Autodesk Inventor part; units mm, degrees
ref_plane "YZ Plane" through (0, 0, 0) normal (1, 0, 0) x (0, 1, 0)
ref_plane "XZ Plane" through (0, 0, 0) normal (0, 1, 0) x (-1, 0, 0)
ref_plane "XY Plane" through (0, 0, 0) normal (0, 0, 1) x (1, 0, 0)
sketch "Skizze1" plane through (0, 0, 0) normal (1, 0, 0) x (0, 1, 0)
  line L0 (-10, -10) -> (-10, -5)
  line L1 (-10, -5) -> (-15, -5)
  line L2 (-15, -5) -> (-15, 0)
  line L3 (-15, 0) -> (15, 0)
  line L4 (15, 0) -> (15, -5)
  line L5 (15, -5) -> (10, -5)
  line L6 (10, -5) -> (10, -10)
  line L7 (10, -10) -> (20, -10)
  line L8 (20, -10) -> (20, -30)
  line L9 (20, -30) -> (-20, -30)
  line L10 (-20, -30) -> (-20, -10)
  line L11 (-20, -10) -> (-10, -10)
  line L12 (0, -36) -> (0, 6)
  point P0 (0, 0)
  dimension "d0" = 30
  dimension "d1" = 20
  dimension "d2" = 5
  dimension "d3" = 5
  dimension "d4" = 20
  dimension "d5" = 90
  dimension "d6" = 40
extrude "Extrusion1" add sketch "Skizze1" along normal blind 10
sketch "Skizze3" plane through (0, 20, -10) normal (0, 1, 0) x (1, 0, 0)
  line L0 (0, 0) -> (0, 20)
  line L1 (0, 20) -> (40, 20)
  line L2 (40, 20) -> (40, 80)
  line L3 (40, 80) -> (-10, 80)
  line L4 (-10, 80) -> (-10, 90)
  line L5 (-10, 90) -> (50, 90)
  line L6 (50, 90) -> (50, 10)
  line L7 (50, 10) -> (0, 10)
  point P0 (0, -10)
  dimension "d12" = 10
  dimension "d13" = 10
  dimension "d14" = 10
  dimension "d15" = 60
  dimension "d16" = 50
  dimension "d17" = 60
extrude "Extrusion3" add sketch "Skizze3" against normal up to surface (40 mm away)
sketch "Skizze4" plane through (50, 20, -100) normal (0, 0, -1) x (-1, 0, 0)
  arc A0 (53.3975, 30) -> (53.3975, -70) centre (140, -20) ccw
  arc A1 (62.0577, 25) -> (62.0577, -65) centre (140, -20) ccw
  line L0 (140, -20) -> (53.3975, -70)
  line L1 (140, -20) -> (53.3975, 30)
  line L2 (0, -40) -> (60, -40)
  line L3 (0, 0) -> (60, 0)
  line L4 (0, 0) -> (0, -40)
  point P0 (40, -20)
  point P1 (42.0204, 0)
  point P2 (52.2504, 0)
  point P3 (52.2504, -40)
  point P4 (42.0204, -40)
  dimension "d20" = 200
  dimension "d21" = 180
  dimension "d22" = 30
  dimension "d23" = 30
  dimension "d24" = 40
  dimension "d25" = 20
  dimension "d30" = 140
extrude "Extrusion4" add sketch "Skizze4" against normal up to surface (10 mm away) contours L1 A1 L3 A0 | L2 A1 L0 A0
sketch "Skizze5" plane through (40, -20, -90) normal (0, 0, 1) x (1, 0, 0)
  arc A0 (-42.2504, 40) -> (-52.0577, 65) centre (-130, 20) ccw
  circle A1 centre (-130, 20) radius 90
  point P0 (-40, 20)
  point P1 (-52.0577, 65)
  point P2 (-42.2504, 40)
extrude "Extrusion5" cut sketch "Skizze5" against normal up to surface (10 mm away)
sketch "Skizze6" plane through (40, -20, -90) normal (0, 0, 1) x (1, 0, 0)
  arc A0 (-52.0577, -25) -> (-52.0577, 65) centre (-130, 20) ccw
  line L0 (-43.3975, -30) -> (-52.0577, -25)
  arc A1 (-43.3975, -30) -> (-32.0204, 0) centre (-130, 20) ccw
  line L1 (-32.0204, 0) -> (0, 0)
  line L2 (0, 40) -> (0, 0)
  line L3 (-32.0204, 40) -> (0, 40)
  arc A2 (-32.0204, 40) -> (-43.3975, 70) centre (-130, 20) ccw
  line L4 (-52.0577, 65) -> (-43.3975, 70)
  line L5 (-30, 0) -> (-30, 40)
  line L6 (-30, 0) -> (10, 0)
  line L7 (10, 40) -> (10, 0)
  line L8 (-30, 40) -> (10, 40)
  point P0 (-40, 20)
extrude "Extrusion6" cut sketch "Skizze6" along normal through all
equation "\"d13\" = d12"
equation "\"d23\" = d22"
equation "\"d25\" = 0.5 * d24"
properties part number "Finger"
Could you check a few things on this model? Use its own coordinates, in mm. A direction names the side the tool comes from. Round coordinates to 2 decimals unless told otherwise and drop trailing zeros. Loops run counter-clockwise (first coordinate to the right, second up) from the corner with the lowest first, then second, coordinate; pieces in that order, holes last. Notation, with made-up numbers: M -6.75,48.5 L 42.25,48.5 A16 ccw 42.25,63.5 Z; hole C -34,21.5 d5. An arc over 180 degrees is marked long. Put each result on its own line as item: value.
Q1. I need wall thicknesses on probe 1 along Y at (x, z) = (31.5, -93); probe 2 along Y at (x, z) = (-7, -98.5); probe 3 along X at (y, z) = (-1, -93.75). Which ranges of each line are inside material? Lowest first, please.
Check result:
probe 1: -20 to 20
probe 2: -47.92 to -34.8, 34.8 to 47.92
probe 3: -0.01 to 50
Q2. Imagine slicing it at D-D (y = -3). Write out the boundary of the cut face in (x, z), then the cut area to 4 significant figures.
Check result:
outline: M -0.05,-100 L 50,-100 L 50,-90 L -0.05,-90 Z
area: 500.5 mm2
Q3. Imagine slicing it at C-C (x = 32.5). Write out the boundary of the cut face in (y, z).
Check result:
outline: M -20,-100 L 20,-100 L 20,-90 L -20,-90 Z
Q4. For pin 1 (4 mm diameter, centred on x = 32.5, z = -91.5, fed in from -Y); pin 2 (2 mm diameter, centred on y = 22.5, z = -94, fed in from -X), each with a flat end and sliding along its axis, tell me the tip position at first contact or that it passes through.
Check result:
pin 1: y = -20
pin 2: x = -3.12
Q5. Imagine slicing it at A-A (x = -6). Write out the boundary of the cut face in (y, z), then the cut area to 3 significant figures.
Check result:
outline: M -48.5,-100 L -32.31,-100 L -32.31,-90 L -48.5,-90 Z; M 32.31,-100 L 48.5,-100 L 48.5,-90 L 32.31,-90 Z
area: 324 mm2
Q6. Thinking about a two-plate mould opening in Y: for faces 4 (the face through (0, 0, -95)), 5 (the face through (29, 20, -95)), 6 (the face through (-7.788, -47.465, -95.07)), which applies, released by +Y, released by -Y, zero draft, split by the parting line, or undercut?
Check result:
face 4: undercut
face 5: released by +Y
face 6: released by -Y
Q7. Imagine slicing it at B-B (z = -94.5). Write out the boundary of the cut face in (x, y), then the cut area to 3 significant figures.
Check result:
outline: M -12.06,-45 L -3.4,-50 A100 ccw 7.98,-20 L 50,-20 L 50,20 L 7.98,20 A100 ccw -3.4,50 L -12.06,45 A90 cw Z
area: 2,620 mm2
Q8. On a 3-axis mill with a long thin cutter (end or side, diameter ignored), from which of +Z, -Z, +X, -X, +Y, -Y can I reach the whole of each face in a straight line? I mean faces 1 (the face through (-6.148, -32.692, -95.07)), 2 (the face through (29, -20, -95)), 3 (the face through (-7.788, 47.465, -95.07)). Say none if no direction works.
Check result:
face 1: +Z, -Z, -X
face 2: +Z, -Z, +X, -Y
face 3: +Z, -Z, -X, +Y
